```python
from build123d import *

# Parameters (mm, degrees)
F0_W          = 31
F0_H          = 24
F1_DEPTH      = 3
F3_DEPTH      = 16.5
F5_DEPTH      = 2
F6_W          = 2
F6_H          = 4
F7_DEPTH      = 8
F7_DEPTH_BACK = 15
F8_SIZE       = 0.99999


# Not quite as in the source:
# - a fillet or chamfer is up to 0.001 mm smaller than in the source, because OpenCascade refuses the exact size


with BuildPart() as f1:
    # F0 (on Front) → F1 (new body)
    with BuildSketch(Plane.XZ):
        Rectangle(F0_W, F0_H)
        with BuildLine():
            Line((10, -8.3), (-10, -8.3))
            ThreePointArc((-10, -8.3), (-11.4142135624, -7.7142135624), (-12, -6.3))
            Line((-12, -6.3), (-12, 3.3))
            Line((-12, 3.3), (-7, 8.3))
            Line((-7, 8.3), (7, 8.3))
            Line((7, 8.3), (12, 3.3))
            Line((12, 3.3), (12, -6.3))
            ThreePointArc((12, -6.3), (11.4142135624, -7.7142135624), (10, -8.3))
        make_face(mode=Mode.SUBTRACT)
    extrude(amount=F1_DEPTH)

    # F2 (on face) → F3 (join)
    with BuildSketch(Plane(origin=(0, 0, 0), x_dir=(-1, 0, 0), z_dir=(0, 1, 0))):
        Polygon((-7.5591883092, 9.65), (-13.35, 3.8591883092), (-13.35, -9.65), (13.35, -9.65), (13.35, 3.8591883092), (7.5591883092, 9.65), align=None)
        with BuildLine():
            Line((-12, -6.3), (-12, 3.3))
            Line((-12, 3.3), (-7, 8.3))
            Line((-7, 8.3), (7, 8.3))
            Line((7, 8.3), (12, 3.3))
            Line((12, 3.3), (12, -6.3))
            ThreePointArc((12, -6.3), (11.4142135624, -7.7142135624), (10, -8.3))
            Line((10, -8.3), (-10, -8.3))
            ThreePointArc((-10, -8.3), (-11.4142135624, -7.7142135624), (-12, -6.3))
        make_face(mode=Mode.SUBTRACT)
    extrude(amount=F3_DEPTH)

    # F4 (on face) → F5 (join)
    with BuildSketch(Plane(origin=(0, 16.5, 0), x_dir=(-1, 0, 0), z_dir=(0, 1, 0))):
        Polygon((7.5591883092, 9.65), (-7.5591883092, 9.65), (-13.35, 3.8591883092), (-13.35, -9.65), (13.35, -9.65), (13.35, 3.8591883092), align=None)
    extrude(amount=-F5_DEPTH)

    # F6 (on face) → F7 (join, two sides)
    with BuildSketch(Plane(origin=(0, 16.5, 0), x_dir=(-1, 0, 0), z_dir=(0, 1, 0))) as f7_sk:
        with Locations((0, 4)):
            Rectangle(F6_W, F6_H)
        with Locations((7, -4)):
            Rectangle(F6_W, F6_H)
        with Locations((-7, -4)):
            Rectangle(F6_W, F6_H)
    extrude(amount=F7_DEPTH)
    extrude(f7_sk.sketch, amount=-F7_DEPTH_BACK)

    # F8 (size 1 in the source; OpenCascade refuses exactly that, so slightly less here)
    f8_edges = [f1.edges().sort_by_distance(p)[0] for p in [
        (0, 1.5, 2),
        (-1, 1.5, 4),
        (0, 1.5, 6),
        (1, 1.5, 4),
        (8, 1.5, -4),
        (7, 1.5, -6),
        (6, 1.5, -4),
        (7, 1.5, -2),
        (-7, 1.5, -6),
        (-8, 1.5, -4),
        (-7, 1.5, -2),
        (-6, 1.5, -4),
    ]]
    chamfer(f8_edges, length=F8_SIZE)


solid = f1.part
```
Input: part model. Units: mm. Frame: model coordinates. A direction names the side the tool comes from. Coordinates: 2 decimals unless noted, no trailing zeros. Write each loop counter-clockwise with the first axis right and the second up, starting at its lowest first coordinate (ties: lowest second). Pieces come first, ordered by that corner, then holes. Notation, with made-up numbers: (57.5, -34) -> (62.5, -34) arc R12 cw to (62.5, -11) -> close; hole circle Ø1 at (-32.5, -31). An arc over 180 degrees is marked (long way). Write each question's results on one line, items separated by ' | '.
Item 1: Section query A-A on y = 23.25. Return loops of the section in (x, z), plus the area to 3 significant figures.
Conclusion:
outline: (-8, -6) -> (-6, -6) -> (-6, -2) -> (-8, -2) -> close; (-1, 2) -> (1, 2) -> (1, 6) -> (-1, 6) -> close; (6, -6) -> (8, -6) -> (8, -2) -> (6, -2) -> close | area: 24.0 mm^2
Item 2: Material intervals for probe 1 along X at (y, z) = (1.75, -1.75); probe 2 along Z at (x, y) = (0.5, 5.5); probe 3 along Z at (x, y) = (2, 0.75), sorted ascending.
Conclusion:
probe 1: x = -13.35 to -12, 12 to 13.35 | probe 2: z = -9.65 to -8.3, 2 to 6, 8.3 to 9.65 | probe 3: z = -9.65 to -8.3, 8.3 to 9.65
Item 3: Section query B-B on y = 12.75. Return loops of the section in (x, z), plus the area to 3 significant figures.
Conclusion:
outline: (-13.35, -9.65) -> (13.35, -9.65) -> (13.35, 3.86) -> (7.56, 9.65) -> (-7.56, 9.65) -> (-13.35, 3.86) -> close; (-8, -6) -> (-6, -6) -> (-6, -2) -> (-8, -2) -> close; (-1, 2) -> (1, 2) -> (1, 6) -> (-1, 6) -> close; (6, -6) -> (8, -6) -> (8, -2) -> (6, -2) -> close; hole (-12, -6.3) arc R2 ccw to (-10, -8.3) -> (10, -8.3) arc R2 ccw to (12, -6.3) -> (12, 3.3) -> (7, 8.3) -> (-7, 8.3) -> (-12, 3.3) -> close | area: 134 mm^2
Item 4: Pin query (flat end, axial travel): pin 1 Ø2 at (x, y) = (-7.5, 6.5) entering from +Z; pin 2 Ø2 at (y, z) = (9.5, 4) entering from +X; pin 3 Ø11 at (y, z) = (12.5, -2.5) entering from -X. Return the tip coordinate at first contact, or that it passes through.
Conclusion:
pin 1: stops at z = 9.65 | pin 2: stops at x = 13.35 | pin 3: stops at x = -13.35
Item 5: Set-up query: faces 1 (the flat face through (-7, 20, -6)), 2 (the flat face through (7, 20, -2)), 3 (the flat face through (0, -3, 11)), 4 (the flat face through (8, 9, -4)). Return all of +Z, -Z, +X, -X, +Y, -Y with unobstructed straight access to the full face (end or side cutting, diameter ignored); none if empty.
Conclusion:
face 1: -Z, +X, -X, +Y | face 2: +Z, +X, -X, +Y | face 3: +Z, -Z, +X, -X, -Y | face 4: -Y
Item 6: Section query D-D on x = -3.5. Return loops of the section in (y, z).
Conclusion:
outline: (-3, -12) -> (0, -12) -> (0, -9.65) -> (16.5, -9.65) -> (16.5, 9.65) -> (0, 9.65) -> (0, 12) -> (-3, 12) -> (-3, 8.3) -> (14.5, 8.3) -> (14.5, -8.3) -> (-3, -8.3) -> close
Item 7: Mould query, pull axis X, two halves, no side actions, for faces 5 (the flat face through (-7, 20, -2)), 6 (the flat face through (0, 2.1, 5.6)), 7 (the flat face through (-8, 20, -4)), 8 (the flat face through (1, 20, 4)). Classes: +X half, -X half, draft (parallel to the pull), parting line (faces both ways), or undercut.
Conclusion:
face 5: draft | face 6: undercut | face 7: -X half | face 8: +X half
